Geometry: final body of the model. Coordinates: model frame, mm. Round coordinates to 2 decimals unless told otherwise and drop trailing zeros. Write each loop counter-clockwise with the first axis right and the second up, starting at its lowest first coordinate (ties: lowest second). Pieces come first, ordered by that corner, then holes. Notation, with made-up numbers: M -11.75,79.25 L 24.25,79.25 A22 cw 24.25,98.25 Z; hole C 70,-3.5 d10. An arc over 180 degrees is marked long. Use one line per item in the form item = value. Start each with the question number.
from build123d import *

# Parameters (mm, degrees)
BOSS_EXTRUDE1_DEPTH     = 1.5
SKETCH2_OUTSIDE_W       = 14.11
SKETCH2_OUTSIDE_H       = 5.61
CUT_EXTRUDE1_DEPTH      = 1
CUT_EXTRUDE1_DEPTH_BACK = 4
CUT_EXTRUDE2_DEPTH      = 0.5


with BuildPart() as part:
    # Sketch1 → Boss-Extrude1 (new body, symmetric)
    with BuildSketch(Plane.XY):
        Polygon((0, 0), (10, 1), (10, -0.5), (0, -0.5), align=None)
    extrude(amount=BOSS_EXTRUDE1_DEPTH, both=True)

    # Sketch2 outside → Cut-Extrude1 (cut, two sides)
    with BuildSketch(Plane.XY.offset(1.5)) as cut_extrude1_sk:
        with Locations((5, 0.25)):
            Rectangle(SKETCH2_OUTSIDE_W, SKETCH2_OUTSIDE_H)
        with BuildLine():
            Line((9.816696972, -0.44), (9.766696972, -0.44))
            ThreePointArc((9.766696972, -0.44), (9.675045458, -0.5), (9.583393944, -0.44))
            Line((9.583393944, -0.44), (9.533393944, -0.44))
            ThreePointArc((9.533393944, -0.44), (9.441742431, -0.5), (9.350090917, -0.44))
            Line((9.350090917, -0.44), (9.300090917, -0.44))
            ThreePointArc((9.300090917, -0.44), (9.208439403, -0.5), (9.116787889, -0.44))
            Line((9.116787889, -0.44), (9.066787889, -0.44))
            ThreePointArc((9.066787889, -0.44), (8.975136375, -0.5), (8.883484861, -0.44))
            Line((8.883484861, -0.44), (8.833484861, -0.44))
            ThreePointArc((8.833484861, -0.44), (8.741833347, -0.5), (8.650181833, -0.44))
            Line((8.650181833, -0.44), (8.600181833, -0.44))
            ThreePointArc((8.600181833, -0.44), (8.508530319, -0.5), (8.416878805, -0.44))
            Line((8.416878805, -0.44), (8.366878805, -0.44))
            ThreePointArc((8.366878805, -0.44), (8.275227292, -0.5), (8.183575778, -0.44))
            Line((8.183575778, -0.44), (8.133575778, -0.44))
            ThreePointArc((8.133575778, -0.44), (8.041924264, -0.5), (7.95027275, -0.44))
            Line((7.95027275, -0.44), (7.90027275, -0.44))
            ThreePointArc((7.90027275, -0.44), (7.808621236, -0.5), (7.716969722, -0.44))
            Line((7.716969722, -0.44), (7.666969722, -0.44))
            ThreePointArc((7.666969722, -0.44), (7.575318208, -0.5), (7.483666694, -0.44))
            Line((7.483666694, -0.44), (7.433666694, -0.44))
            ThreePointArc((7.433666694, -0.44), (7.34201518, -0.5), (7.250363666, -0.44))
            Line((7.250363666, -0.44), (7.200363666, -0.44))
            ThreePointArc((7.200363666, -0.44), (7.108712153, -0.5), (7.017060639, -0.44))
            Line((7.017060639, -0.44), (6.967060639, -0.44))
            ThreePointArc((6.967060639, -0.44), (6.875409125, -0.5), (6.783757611, -0.44))
            Line((6.783757611, -0.44), (6.733757611, -0.44))
            ThreePointArc((6.733757611, -0.44), (6.642106097, -0.5), (6.550454583, -0.44))
            Line((6.550454583, -0.44), (6.500454583, -0.44))
            ThreePointArc((6.500454583, -0.44), (6.408803069, -0.5), (6.317151555, -0.44))
            Line((6.317151555, -0.44), (6.267151555, -0.44))
            ThreePointArc((6.267151555, -0.44), (6.175500041, -0.5), (6.083848527, -0.44))
            Line((6.083848527, -0.44), (6.033848527, -0.44))
            ThreePointArc((6.033848527, -0.44), (5.942197014, -0.5), (5.8505455, -0.44))
            Line((5.8505455, -0.44), (5.8005455, -0.44))
            ThreePointArc((5.8005455, -0.44), (5.708893986, -0.5), (5.617242472, -0.44))
            Line((5.617242472, -0.44), (5.567242472, -0.44))
            ThreePointArc((5.567242472, -0.44), (5.475590958, -0.5), (5.383939444, -0.44))
            Line((5.383939444, -0.44), (5.333939444, -0.44))
            ThreePointArc((5.333939444, -0.44), (5.24228793, -0.5), (5.150636416, -0.44))
            Line((5.150636416, -0.44), (5.100636416, -0.44))
            ThreePointArc((5.100636416, -0.44), (5.008984902, -0.5), (4.917333388, -0.44))
            Line((4.917333388, -0.44), (4.867333388, -0.44))
            ThreePointArc((4.867333388, -0.44), (4.775681875, -0.5), (4.684030361, -0.44))
            Line((4.684030361, -0.44), (4.634030361, -0.44))
            ThreePointArc((4.634030361, -0.44), (4.542378847, -0.5), (4.450727333, -0.44))
            Line((4.450727333, -0.44), (4.400727333, -0.44))
            ThreePointArc((4.400727333, -0.44), (4.309075819, -0.5), (4.217424305, -0.44))
            Line((4.217424305, -0.44), (4.167424305, -0.44))
            ThreePointArc((4.167424305, -0.44), (4.075772791, -0.5), (3.984121277, -0.44))
            Line((3.984121277, -0.44), (3.934121277, -0.44))
            ThreePointArc((3.934121277, -0.44), (3.842469763, -0.5), (3.750818249, -0.44))
            Line((3.750818249, -0.44), (3.700818249, -0.44))
            ThreePointArc((3.700818249, -0.44), (3.609166736, -0.5), (3.517515222, -0.44))
            Line((3.517515222, -0.44), (3.467515222, -0.44))
            ThreePointArc((3.467515222, -0.44), (3.375863708, -0.5), (3.284212194, -0.44))
            Line((3.284212194, -0.44), (3.234212194, -0.44))
            ThreePointArc((3.234212194, -0.44), (3.14256068, -0.5), (3.050909166, -0.44))
            Line((3.050909166, -0.44), (3.000909166, -0.44))
            ThreePointArc((3.000909166, -0.44), (2.909257652, -0.5), (2.817606138, -0.44))
            Line((2.817606138, -0.44), (2.767606138, -0.44))
            ThreePointArc((2.767606138, -0.44), (2.675954624, -0.5), (2.58430311, -0.44))
            Line((2.58430311, -0.44), (2.53430311, -0.44))
            ThreePointArc((2.53430311, -0.44), (2.442651597, -0.5), (2.351000083, -0.44))
            Line((2.351000083, -0.44), (2.301000083, -0.44))
            ThreePointArc((2.301000083, -0.44), (2.209348569, -0.5), (2.117697055, -0.44))
            Line((2.117697055, -0.44), (2.067697055, -0.44))
            ThreePointArc((2.067697055, -0.44), (1.976045541, -0.5), (1.884394027, -0.44))
            Line((1.884394027, -0.44), (1.834394027, -0.44))
            ThreePointArc((1.834394027, -0.44), (1.742742513, -0.5), (1.651090999, -0.44))
            Line((1.651090999, -0.44), (1.601090999, -0.44))
            ThreePointArc((1.601090999, -0.44), (1.509439485, -0.5), (1.417787971, -0.44))
            Line((1.417787971, -0.44), (1.367787971, -0.44))
            ThreePointArc((1.367787971, -0.44), (1.276136458, -0.5), (1.184484944, -0.44))
            Line((1.184484944, -0.44), (1.134484944, -0.44))
            ThreePointArc((1.134484944, -0.44), (1.04283343, -0.5), (0.951181916, -0.44))
            Line((0.951181916, -0.44), (0.901181916, -0.44))
            ThreePointArc((0.901181916, -0.44), (0.809530402, -0.5), (0.717878888, -0.44))
            Line((0.717878888, -0.44), (0.667878888, -0.44))
            ThreePointArc((0.667878888, -0.44), (0.576227374, -0.5), (0.48457586, -0.44))
            Line((0.48457586, -0.44), (0.43457586, -0.44))
            ThreePointArc((0.43457586, -0.44), (0.342924346, -0.5), (0.251272832, -0.44))
            Line((0.251272832, -0.44), (0.201272832, -0.44))
            ThreePointArc((0.201272832, -0.44), (0.109621319, -0.5), (0.017969805, -0.44))
            Line((0.017969805, -0.44), (0, -0.44))
            Line((0, -0.44), (0, 0))
            Line((0, 0), (10, 1))
            Line((10, 1), (10, -0.44))
            ThreePointArc((10, -0.44), (9.908348486, -0.5), (9.816696972, -0.44))
        make_face(mode=Mode.SUBTRACT)
    extrude(amount=CUT_EXTRUDE1_DEPTH, mode=Mode.SUBTRACT)
    extrude(cut_extrude1_sk.sketch, amount=-CUT_EXTRUDE1_DEPTH_BACK, mode=Mode.SUBTRACT)

    # Sketch4 → Cut-Extrude2 (cut)
    with BuildSketch(Plane(origin=(10, 0, 0), x_dir=(0, 0, -1), z_dir=(1, 0, 0))):
        Polygon((-1.5, -0.5), (1.5, -0.5), (1.5, -0.44), (1.5, 1), (-1.5, 1), (-1.500006, -0.44), align=None)
    extrude(amount=-CUT_EXTRUDE2_DEPTH, mode=Mode.SUBTRACT)


solid = part.part
1. Section query B-B (x = 8.5). Return loops of the section in (y, z), then the cut area to 3 significant figures.
2. Section query A-A (y = 0.3). Return loops of the section in (x, z), then the cut area to 3 significant figures.
3. Ray query, probe 1 along Y at (x, z) = (2, -1.1); probe 2 along Y at (x, z) = (5.5, -1.2). Return the intervals inside material, ascending.
Checks:
q1.outline = M -0.5,-1.5 L 0.85,-1.5 L 0.85,1.5 L -0.5,1.5 Z
q1.area = 4.05 mm^2
q2.outline = M 3,-1.5 L 9.5,-1.5 L 9.5,1.5 L 3,1.5 Z
q2.area = 19.5 mm^2
q3.probe_1 = -0.5 to 0.2
q3.probe_2 = -0.5 to 0.55
